Source: CAD feature listing. Evaluate the final solid. Frame: model axes, mm. Face numbers are marked on the shaded views. A direction names the side the tool comes from. Round coordinates to 2 decimals unless told otherwise and drop trailing zeros. Loops run counter-clockwise (first coordinate to the right, second up) from the corner with the lowest first, then second, coordinate; pieces in that order, holes last. Notation, with made-up numbers: M 26.5,14.5 L 53.5,14.5 A27 cw 53.5,30.5 Z; hole C -22.75,8 d4. An arc over 180 degrees is marked long. Answer as a JSON object with one key per item and string values.
from build123d import *

# Parameters (mm, degrees)
BOSS_EXTRUDE1_DEPTH = 60
SKETCH3_W           = 20
SKETCH3_H           = 20
CUT_EXTRUDE1_DEPTH  = 1040.5
CUT_EXTRUDE2_REACH  = 72.077


with BuildPart() as part:
    # Sketch1 → Boss-Extrude1 (new body)
    with BuildSketch(Plane(origin=(0, 0, 0), x_dir=(1, 0, 0), z_dir=(0, 1, 0))):
        with BuildLine():
            Line((2.8, 0), (22.8, 0))
            ThreePointArc((22.8, 0), (24.779898987, -0.820101013), (25.6, -2.8))
            Line((25.6, -2.8), (25.6, -22.8))
            ThreePointArc((25.6, -22.8), (24.779898987, -24.779898987), (22.8, -25.6))
            Line((22.8, -25.6), (2.8, -25.6))
            ThreePointArc((2.8, -25.6), (0.820101013, -24.779898987), (0, -22.8))
            Line((0, -22.8), (0, -2.8))
            ThreePointArc((0, -2.8), (0.820101013, -0.820101013), (2.8, 0))
        make_face()
    extrude(amount=BOSS_EXTRUDE1_DEPTH)

    # Sketch3 → Cut-Extrude1 (cut)
    with BuildSketch(Plane(origin=(0, 0, 0), x_dir=(-1, 0, 0), z_dir=(0, -1, 0))):
        with Locations((-12.8, -12.8)):
            Rectangle(SKETCH3_W, SKETCH3_H)
    extrude(amount=-CUT_EXTRUDE1_DEPTH, mode=Mode.SUBTRACT)

    # Cut-Extrude2: up to this face of the body (flat: up to its plane)
    cut_extrude2_end = Plane(part.part.faces().sort_by_distance((12.8, 30, 0))[0])
    # Sketch4 → Cut-Extrude2 (cut, up to the picked face)
    with BuildSketch(Plane.XY.offset(25.6), mode=Mode.PRIVATE) as cut_extrude2_sk1:
        Polygon((-0.986658786, 35.401585719), (-0.986658786, 60), (27.022015216, 60), (27.022015216, 58.911274466), align=None)
    cut_extrude2_tool1 = split(extrude(cut_extrude2_sk1.sketch, amount=-CUT_EXTRUDE2_REACH, mode=Mode.PRIVATE), bisect_by=cut_extrude2_end, keep=Keep.BOTH, mode=Mode.PRIVATE)
    add(cut_extrude2_tool1.solids().sort_by(Axis((8.745273, 51.785147, 25.6), (0, 0, -1)))[0], mode=Mode.SUBTRACT)


solid = part.part
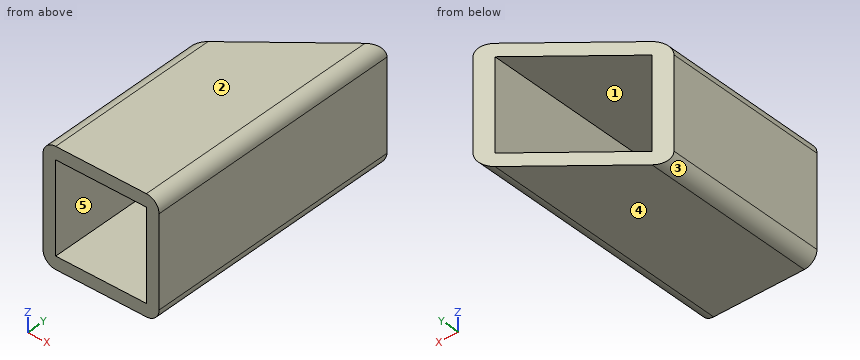
Item 1: Section C-C on y = 6. Return the cut outline in (x, z), then the cut area to 3 significant figures.
Answer sheet:
{"outline": "M 0,2.8 A2.8 ccw 2.8,0 L 22.8,0 A2.8 ccw 25.6,2.8 L 25.6,22.8 A2.8 ccw 22.8,25.6 L 2.8,25.6 A2.8 ccw 0,22.8 Z; hole M 2.8,2.8 L 22.8,2.8 L 22.8,22.8 L 2.8,22.8 Z", "area": "249 mm²"}
Item 2: Access query for the marked faces 1 and 2. Directions: +Z, -Z, +X, -X, +Y, -Y. A direction counts if a zero-diameter tool reaches every point of the face in a straight line with its end or side. Return the directions, or none.
Answer sheet:
{"face 1": "+Y, -Y", "face 2": "+Z, +X, -X, +Y, -Y"}
Item 3: Line query: probe 1 along X at (y, z) = (3.5, 12.5); probe 2 along X at (y, z) = (40, 14.75). Output: solid intervals per line, ascending. Write a range as from..to.
Answer sheet:
{"probe 1": "x = 0..2.8, 22.8..25.6", "probe 2": "x = 22.8..25.6"}
Item 4: Section A-A on z = 8. Return the cut outline in (x, y), then the cut area to 3 significant figures.
Answer sheet:
{"outline": "M 0,0 L 2.8,0 L 2.8,38.58 L 0,36.23 Z; M 22.8,0 L 25.6,0 L 25.6,57.72 L 22.8,55.37 Z", "area": "263 mm²"}
Item 5: Section D-D on y = 46.5. Return the cut outline in (x, z).
Answer sheet:
{"outline": "M 12.24,0 L 22.8,0 A2.8 ccw 25.6,2.8 L 25.6,22.8 A2.8 ccw 22.8,25.6 L 12.24,25.6 L 12.24,22.8 L 22.8,22.8 L 22.8,2.8 L 12.24,2.8 Z"}
Item 6: Section B-B on x = 20. Return the cut outline in (y, z), then the cut area to 3 significant figures.
Answer sheet:
{"outline": "M 0,0 L 53.02,0 L 53.02,2.8 L 0,2.8 Z; M 0,22.8 L 53.02,22.8 L 53.02,25.6 L 0,25.6 Z", "area": "297 mm²"}
Item 7: Contact query for flat-ended pins moving along their axis: pin 1 Ø1 at (y, z) = (50, 13) entering from -X; pin 2 Ø1 at (x, y) = (6.5, 43) entering from +Z; pin 3 Ø1.5 at (x, z) = (22.5, 20) entering from +Y; pin 4 Ø10 at (x, z) = (20.5, 18) entering from +Y. Output: stop coordinate, or through.
Answer sheet:
{"pin 1": "stops at x = 22.8", "pin 2": "passes through", "pin 3": "stops at y = 55.75", "pin 4": "stops at y = 57.63"}
Item 8: Pull-direction query (X, two-part tool) for the marked faces 3, 4 and 5; classes: pulls with the +X half, pulls with the -X half, needs draft (parallel to the pull), parting line crosses it, or undercut.
Answer sheet:
{"face 3": "pulls with the -X half", "face 4": "needs draft", "face 5": "undercut"}
